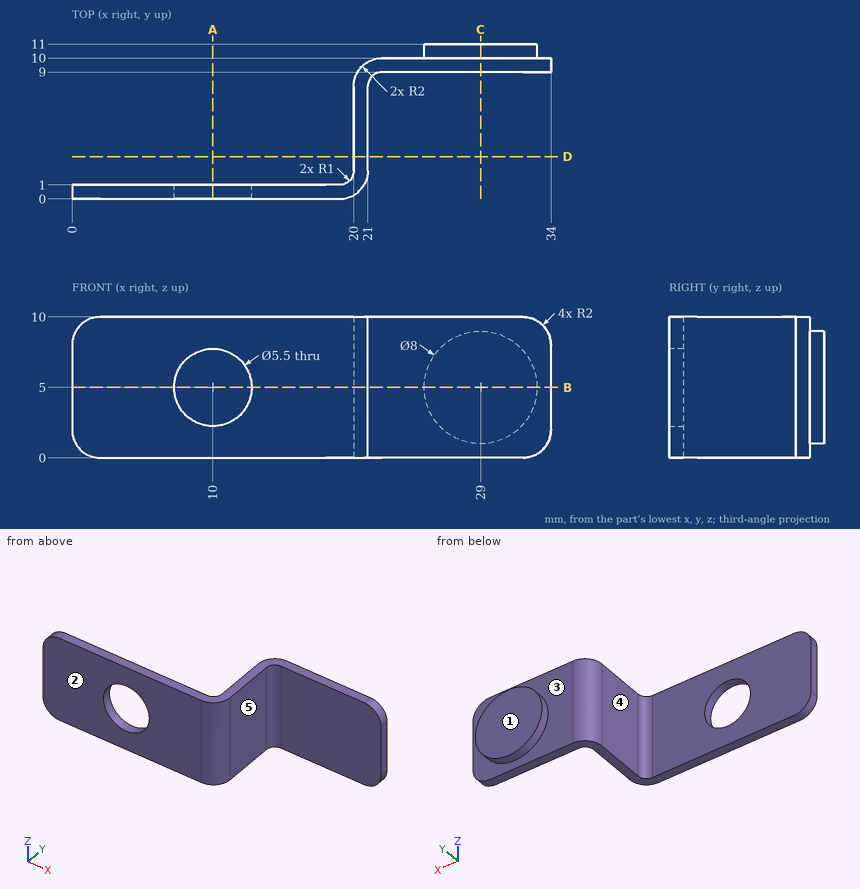
Answer from the drawing. Dimensions are ordinates in mm from the lowest x, y and z of the part. A direction names the side the tool comes from. Coordinates: 2 decimals unless noted, no trailing zeros. Loops run counter-clockwise (first coordinate to the right, second up) from the corner with the lowest first, then second, coordinate; pieces in that order, holes last. Notation, with made-up numbers: (23, -33) -> (53, -33) arc R4 ccw to (53, -28) -> close; hole circle Ø3 at (37.25, -21.75). An arc over 180 degrees is marked (long way). Return JSON: item names as keys, results as strings.
Item 1: Find the intervals of material crossed by probe 1 along Y at (x, z) = (8, 7.5); probe 2 along X at (y, z) = (8, 7.75); probe 3 along X at (y, z) = (0.5, 5), in increasing order.
Answers:
{"probe 1": "y = 0 to 1", "probe 2": "x = 20 to 21", "probe 3": "x = 0 to 7.25, 12.75 to 20.32"}
Item 2: Find section D-D (y = 3). Determine the outline of the cut face in (x, z).
Answers:
{"outline": "(20, 0) -> (21, 0) -> (21, 10) -> (20, 10) -> close"}
Item 3: Find section C-C (x = 29). Determine the outline of the cut face in (y, z).
Answers:
{"outline": "(9, 0) -> (10, 0) -> (10, 1) -> (11, 1) -> (11, 9) -> (10, 9) -> (10, 10) -> (9, 10) -> close"}
Item 4: Find section A-A (x = 10). Determine the outline of the cut face in (y, z), plus the area to 3 significant figures.
Answers:
{"outline": "(0, 0) -> (1, 0) -> (1, 2.25) -> (0, 2.25) -> close; (0, 7.75) -> (1, 7.75) -> (1, 10) -> (0, 10) -> close", "area": "4.50 mm2"}
Item 5: For the marked faces 1, 2, 3, 4 and 5, determine the directions among +Z, -Z, +X, -X, +Y, -Y from which every point of the face is accessible in a straight line to the end or side of a thin tool.
Answers:
{"face 1": "+Z, -Z, +X, -X, +Y", "face 2": "+Z, -Z, +X, -X, -Y", "face 3": "+Y", "face 4": "+Z, -Z, -X, +Y", "face 5": "+Z, -Z, +X, -Y"}
Item 6: Find section B-B (z = 5). Determine the outline of the cut face in (x, y), plus the area to 3 significant figures.
Answers:
{"outline": "(0, 0) -> (7.25, 0) -> (7.25, 1) -> (0, 1) -> close; (12.75, 0) -> (19, 0) arc R2 ccw to (21, 2) -> (21, 8) arc R1 cw to (22, 9) -> (34, 9) -> (34, 10) -> (33, 10) -> (33, 11) -> (25, 11) -> (25, 10) -> (22, 10) arc R2 ccw to (20, 8) -> (20, 2) arc R1 cw to (19, 1) -> (12.75, 1) -> close", "area": "44.2 mm2"}
Item 7: Flat-ended cylindrical pins translate along their axes: P1, Ø6, axis at y = 7.5, z = 4.5, coming from the +X side; P2, Ø3, axis at y = 4.5, z = 2.5, coming from the +X side; P3, Ø3, axis at x = 29, z = 7, coming from the -Y side; P4, Ø1.8, axis at y = 3.5, z = 6, coming from the -X side. Find the tip coordinate at first contact, or state that the pin passes through.
Answers:
{"P1": "stops at x = 34", "P2": "stops at x = 21", "P3": "stops at y = 9", "P4": "stops at x = 20"}
